Source: CAD feature listing. Evaluate the final solid. Frame: model axes, mm. Coordinates: 2 decimals unless noted, no trailing zeros. Write each loop counter-clockwise with the first axis right and the second up, starting at its lowest first coordinate (ties: lowest second). Pieces come first, ordered by that corner, then holes. Notation, with made-up numbers: M 68,7 L 83,7 A18 ccw 83,29 Z; hole C -10.5,70 d8. An arc over 180 degrees is marked long. One line per item, written item: value. Start each with the question number.
Item 1: Cut plane D-D, the plane y = 61.5. Output: boundary loops of the cut face in (x, z) (1 decimal), then the cut area to 3 significant figures.
Item 2: Cut plane A-A, the plane y = 42.5. Output: boundary loops of the cut face in (x, z) (1 decimal).
Item 3: Ray query, L1, parallel to Y at x = 56.5, z = 2.1 (1 decimal); L2, parallel to Y at x = -6, z = 1.85 (1 decimal). Return the intervals inside material, ascending. Write a range as from..to.
Item 4: Cut plane B-B, the plane x = 6. Output: boundary loops of the cut face in (y, z) (1 decimal), then the cut area to 3 significant figures.
Item 5: Cut plane C-C, the plane z = 2.1. Output: boundary loops of the cut face in (x, y) (1 decimal), then the cut area to 3 significant figures.
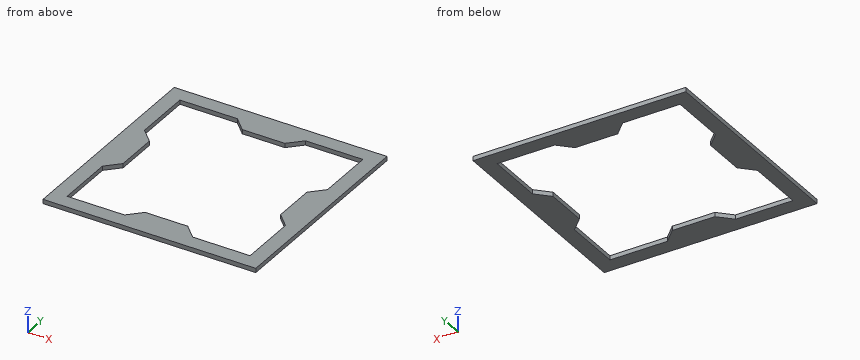
```python
from build123d import *

# Parameters (mm, degrees)
SKETCH1_W           = 158.75
SKETCH1_H           = 158.75
SKETCH1_W_2         = 136.525
SKETCH1_H_2         = 136.525
BOSS_EXTRUDE1_DEPTH = 3.175


with BuildPart() as part:
    # Sketch1 → Boss-Extrude1 (new body)
    with BuildSketch(Plane.XY):
        Rectangle(SKETCH1_W, SKETCH1_H)
        Rectangle(SKETCH1_W_2, SKETCH1_H_2, mode=Mode.SUBTRACT)
        Polygon((25.4, 68.2625), (-25.4, 68.2625), (-15.875, 58.7375), (15.875, 58.7375), align=None)
        Polygon((68.2625, -25.4), (68.2625, 25.4), (58.7375, 15.875), (58.7375, -15.875), align=None)
        Polygon((-15.875, -58.7375), (-25.4, -68.2625), (25.4, -68.2625), (15.875, -58.7375), align=None)
        Polygon((-58.7375, 15.875), (-68.2625, 25.4), (-68.2625, -25.4), (-58.7375, -15.875), align=None)
    extrude(amount=BOSS_EXTRUDE1_DEPTH)


solid = part.part
```
From the geometry:
1. outline: M -79.4,0 L -68.3,0 L -68.3,3.2 L -79.4,3.2 Z; M -18.6,0 L 18.6,0 L 18.6,3.2 L -18.6,3.2 Z; M 68.3,0 L 79.4,0 L 79.4,3.2 L 68.3,3.2 Z
1. area: 189 mm²
2. outline: M -79.4,0 L -68.3,0 L -68.3,3.2 L -79.4,3.2 Z; M 68.3,0 L 79.4,0 L 79.4,3.2 L 68.3,3.2 Z
3. L1: y = -79.4..-68.3, 68.3..79.4
3. L2: y = -79.4..-58.7, 58.7..79.4
4. outline: M -79.4,0 L -58.7,0 L -58.7,3.2 L -79.4,3.2 Z; M 58.7,0 L 79.4,0 L 79.4,3.2 L 58.7,3.2 Z
4. area: 131 mm²
5. outline: M -79.4,-79.4 L 79.4,-79.4 L 79.4,79.4 L -79.4,79.4 Z; hole M -68.3,-68.3 L -25.4,-68.3 L -15.9,-58.7 L 15.9,-58.7 L 25.4,-68.3 L 68.3,-68.3 L 68.3,-25.4 L 58.7,-15.9 L 58.7,15.9 L 68.3,25.4 L 68.3,68.3 L 25.4,68.3 L 15.9,58.7 L -15.9,58.7 L -25.4,68.3 L -68.3,68.3 L -68.3,25.4 L -58.7,15.9 L -58.7,-15.9 L -68.3,-25.4 Z
5. area: 8,140 mm²
